Design review of the part shown in the three views and the two pictorial views. Dimensions are in mm from the part's minimum x, y and z. A direction names the side the tool comes from. Give positions to 0.01 mm unless a question says otherwise; leave off trailing zeros. Loops run counter-clockwise (first coordinate to the right, second up) from the corner with the lowest first, then second, coordinate; pieces in that order, holes last. Notation, with made-up numbers: (-8, 67.5) - (2, 67.5) arc R25 cw to (2, 93.5) - close; hole circle Ø6 at (30.5, -10.75). An arc over 180 degrees is marked (long way). Use CSV: the item, a comma, the result in double quotes. Start each with the question number.
1. For the marked faces 1, 2 and 3, list the 3-axis set-ups (+Z, -Z, +X, -X, +Y, -Y) from which the entire face can be reached by the end or side of a thin tool; tool diameter is ignored.
2. Take a section at C-C on x = 21.25. Give the boundary of the cut face in (y, z), plus the area to 3 significant figures.
3. Mouldability with a two-part tool opening along Y and no side actions: class the marked faces 4, 5, 6 and 7 as pulls with the +Y half, pulls with the -Y half, needs draft (parallel to the pull), parting line crosses it, or undercut.
4. Take a section at B-B on z = 14. Give the boundary of the cut face in (x, y).
5. Take a section at A-A on y = 26.5. Give the boundary of the cut face in (x, z), plus the area to 3 significant figures.
6. Wall thickness on line 1 (Y direction, x = 6.5, z = 21); line 2 (X direction, y = 34, z = 47); line 3 (Z direction, x = 9.5, y = 21): over which ranges is each line inside the solid? List them lowest first.
7. Take a section at D-D on z = 42.5. Give the boundary of the cut face in (x, y).
8. For pin 1 (2 mm diameter, centred on x = 22, z = 17.5, fed in from -Y); pin 2 (2 mm diameter, centred on x = 6.5, y = 22.5, fed in from +Z); pin 3 (3 mm diameter, centred on x = 15, y = 26.5, fed in from -Z), all flat-tipped, find the tip position at first contact; note any pin that passes through.
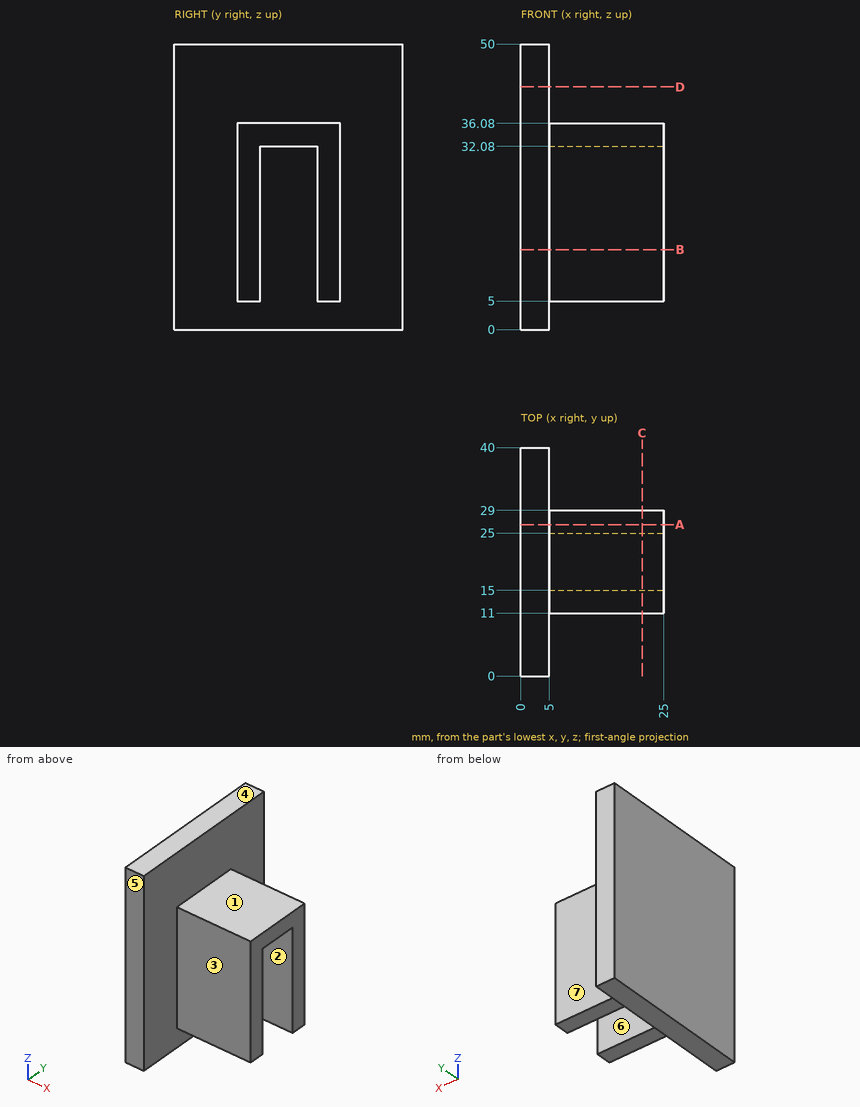
Check result:
1,face 1,"+Z, +X, +Y, -Y"
1,face 2,"-Z, +X"
1,face 3,"+Z, -Z, +X, -Y"
2,outline,"(11, 5) - (15, 5) - (15, 32.08) - (25, 32.08) - (25, 5) - (29, 5) - (29, 36.08) - (11, 36.08) - close"
2,area,"289 mm²"
3,face 4,"needs draft"
3,face 5,"pulls with the -Y half"
3,face 6,"undercut"
3,face 7,"pulls with the +Y half"
4,outline,"(0, 0) - (5, 0) - (5, 11) - (25, 11) - (25, 15) - (5, 15) - (5, 25) - (25, 25) - (25, 29) - (5, 29) - (5, 40) - (0, 40) - close"
5,outline,"(0, 0) - (5, 0) - (5, 5) - (25, 5) - (25, 36.08) - (5, 36.08) - (5, 50) - (0, 50) - close"
5,area,"872 mm²"
6,line 1,"y = 11 to 15, 25 to 29"
6,line 2,"x = 0 to 5"
6,line 3,"z = 32.08 to 36.08"
7,outline,"(0, 0) - (5, 0) - (5, 40) - (0, 40) - close"
8,pin 1,"stops at y = 11"
8,pin 2,"stops at z = 36.08"
8,pin 3,"stops at z = 5"
